Check sheet for the modelled part. Datum: model origin and axes. Units: mm. Face numbers are marked on the shaded views. A direction names the side the tool comes from. Give positions to 0.01 mm unless a question says otherwise; leave off trailing zeros. Write each loop counter-clockwise with the first axis right and the second up, starting at its lowest first coordinate (ties: lowest second). Pieces come first, ordered by that corner, then holes. Notation, with made-up numbers: (-37.75, 6.25) -> (5.25, 6.25) arc R32 cw to (5.25, 44.25) -> close; hole circle Ø11 at (-25.75, 16.5). An arc over 180 degrees is marked (long way). Use a Markdown table: item, result. Add a question column.
1. Cross-section at C-C (z = 12.5). Enter the section's corners in (x, y), then the cut area to 3 significant figures.
2. Cross-section at B-B (x = 15). Enter the section's corners in (y, z).
3. Scan lines: probe 1 along X at (y, z) = (22, 12.5); probe 2 along Y at (x, z) = (-5, 43); probe 3 along Y at (x, z) = (13, 44.5). Record each from-to range of solid material in increasing order. Write a range as [from, to].
4. Cross-section at A-A (z = 29). Enter the section's corners in (x, y).
5. Cross-section at D-D (x = -3). Enter the section's corners in (y, z).
6. Gauge pin test, flat ends, axial feed: P1, Ø7, axis at y = 15, z = 16.5, coming from the -X side; P2, Ø5, axis at x = -6, z = 8, coming from the +Y side; P3, Ø5, axis at x = 3, y = -2.5, coming from the +Z side; P4, Ø7.5, axis at y = 8.5, z = 54.5, coming from the +X side. Record the tip position at first contact, or that the pin passes through.
7. Release check for a two-part mould opening along Y. For the marked faces 6, 7 and 8 record: released by +Y, released by -Y, zero draft, split by the parting line, or undercut.
8. Set-up check for the marked faces 1, 2, 3, 4 and 5: record each of +Z, -Z, +X, -X, +Y, -Y from which the full face is reachable in a straight line by a thin tool's end or side.
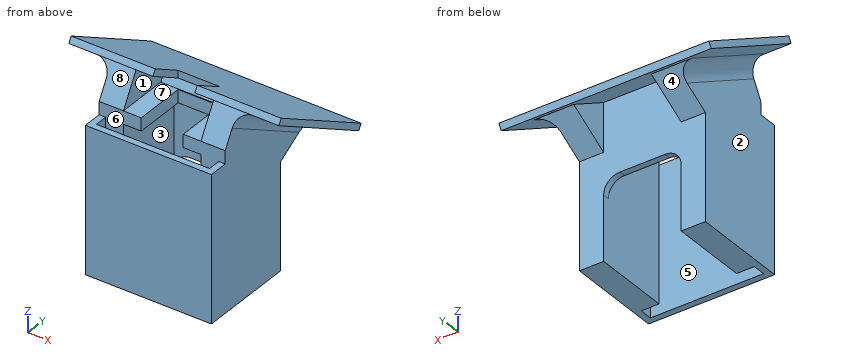
from build123d import *

# Parameters (mm, degrees)
EXTRUDE_1_DEPTH          = 45
EXTRUDE_2_DEPTH          = 4
SKETCH_3_W               = 24
SKETCH_3_H               = 2
CUT_EXTRUDE_1_DEPTH      = 25
SKETCH_5_W               = 40
SKETCH_5_H               = 65
EXTRUDE_3_DEPTH          = 1
CUT_EXTRUDE_2_DEPTH      = 72.51497427
CUT_EXTRUDE_2_DEPTH_BACK = 72.51497427
SKETCH_6_W               = 13
SKETCH_6_H               = 16
EXTRUDE_6_DEPTH          = 2
EXTRUDE_7_DEPTH          = 2
EXTRUDE_8_DEPTH          = 2
EXTRUDE_9_DEPTH          = 2
FILLET_1_R               = 5
EXTRUDE_10_DEPTH         = 5.5
EXTRUDE_11_DEPTH         = 5.5
SKETCH_18_W              = 24
SKETCH_18_H              = 5
EXTRUDE_13_DEPTH         = 3
FILLET_2_R               = 5


with BuildPart() as part:
    # Sketch 1 → Extrude 1 (new body)
    with BuildSketch(Plane.XY):
        Polygon((-14, 24), (-14, 2), (-19.5, 2), (-19.5, -6), (19.5, -6), (19.5, 2), (14, 2), (14, 24), align=None)
        Polygon((-12, 0), (-12, 22), (12, 22), (12, 0), (17.5, 0), (17.5, -4), (-17.5, -4), (-17.5, 0), align=None, mode=Mode.SUBTRACT)
    extrude(amount=EXTRUDE_1_DEPTH)

    # Sketch 2 → Extrude 2 (add)
    with BuildSketch(Plane.XY.offset(45)):
        Polygon((-14, 24), (-14, 0), (-6.5, 0), (-6.5, 16), (6.5, 16), (6.5, 0), (14, 0), (14, 24), align=None)
    extrude(amount=EXTRUDE_2_DEPTH)

    # Sketch 3 → Cut-Extrude 1 (cut)
    with BuildSketch(Plane(origin=(0, 0, 0), x_dir=(-1, 0, 0), z_dir=(0, 0, -1))):
        with Locations((0, 23)):
            Rectangle(SKETCH_3_W, SKETCH_3_H)
    extrude(amount=-CUT_EXTRUDE_1_DEPTH, mode=Mode.SUBTRACT)



with BuildPart() as body_2:
    # Sketch 5 → Extrude 3 (new, symmetric)
    with BuildSketch(Plane(origin=(0, 27.217622393, 47.142304845), x_dir=(0, -0.8660254037844413, 0.4999999999999954), z_dir=(0, 0.4999999999999954, 0.8660254037844413))):
        with Locations((5, 0)):
            Rectangle(SKETCH_5_W, SKETCH_5_H)
    extrude(amount=EXTRUDE_3_DEPTH, both=True)

    # Sketch 6 → Cut-Extrude 2 (cut, two sides: drawn at the far end of the back side and taken through both)
    with BuildSketch(Plane.XY.offset(49).offset(-CUT_EXTRUDE_2_DEPTH_BACK)):
        with Locations((0, 8)):
            Rectangle(SKETCH_6_W, SKETCH_6_H)
    extrude(amount=CUT_EXTRUDE_2_DEPTH + CUT_EXTRUDE_2_DEPTH_BACK, mode=Mode.SUBTRACT)


with BuildPart() as part_1:
    add(part.part)

    add(body_2.part)  # Extrude 6 merges body 2
    # Sketch 11 → Extrude 6 (add)
    with BuildSketch(Plane.ZY.offset(14)):
        Polygon((40.345299462, 36.990381057), (32.845299462, 24), (47.845299462, 24), align=None)
    extrude(amount=-EXTRUDE_6_DEPTH)

    # Sketch 12 → Extrude 7 (add)
    with BuildSketch(Plane(origin=(14, 0, 0), x_dir=(0, 0, -1), z_dir=(1, 0, 0))):
        Polygon((-47.845299462, 24), (-32.845299462, 24), (-40.345299462, 36.990381057), align=None)
    extrude(amount=-EXTRUDE_7_DEPTH)

    # Sketch 13 → Extrude 8 (add)
    with BuildSketch(Plane.ZY.offset(14)):
        Polygon((49, 22), (49, 0), (58.526279442, 5.5), align=None)
    extrude(amount=-EXTRUDE_8_DEPTH)

    # Sketch 14 → Extrude 9 (add)
    with BuildSketch(Plane(origin=(14, 0, 0), x_dir=(0, 0, -1), z_dir=(1, 0, 0))):
        Polygon((-49, 22), (-49, 0), (-58.526279442, 5.5), align=None)
    extrude(amount=-EXTRUDE_9_DEPTH)

    # Fillet 1
    fillet_1_edges = [part_1.edges().sort_by_distance(p)[0] for p in [
        (12, 23, 25),
        (-12, 23, 25),
    ]]
    fillet(fillet_1_edges, radius=FILLET_1_R)

    # Sketch 16 → Extrude 10 (add)
    with BuildSketch(Plane.ZY.offset(14)):
        Polygon((0, 24), (0, 2), (45, 2), (45, 0), (49, 0), (58.526279442, 5.5), (40.345299462, 36.990381057), (32.845299462, 24), align=None)
    extrude(amount=EXTRUDE_10_DEPTH)

    # Sketch 17 → Extrude 11 (add)
    with BuildSketch(Plane(origin=(14, 0, 0), x_dir=(0, 0, -1), z_dir=(1, 0, 0))):
        Polygon((0, 24), (0, 2), (-45, 2), (-45, 0), (-49, 0), (-58.526279442, 5.5), (-40.345299462, 36.990381057), (-32.845299462, 24), align=None)
    extrude(amount=EXTRUDE_11_DEPTH)

    # Sketch 18 → Extrude 13 (add)
    with BuildSketch(Plane(origin=(0, 26.717622393, 46.276279442), x_dir=(-1, 0, 0), z_dir=(0, -0.4999999999999954, -0.8660254037844414))):
        with Locations((0, -7.947441117)):
            Rectangle(SKETCH_18_W, SKETCH_18_H)
    extrude(amount=EXTRUDE_13_DEPTH)

    # Fillet 2
    fillet_2_edges = [part_1.edges().sort_by_distance(p)[0] for p in [
        (-19.5, 21.245190528, 49.435789452),
        (19.5, 21.245190528, 49.435789452),
    ]]
    fillet(fillet_2_edges, radius=FILLET_2_R)


solid = part_1.part
Worked answers:
| question | item | result |
|---|---|---|
| 1 | outline | (-19.5, -6) -> (19.5, -6) -> (19.5, 24) -> (12, 24) -> (12, 0) -> (17.5, 0) -> (17.5, -4) -> (-17.5, -4) -> (-17.5, 0) -> (-12, 0) -> (-12, 24) -> (-19.5, 24) -> close |
| 1 | area | 454 mm² |
| 2 | outline | (-6, 0) -> (-4, 0) -> (-4, 45) -> (-6, 45) -> close; (0, 0) -> (24, 0) -> (24, 32.85) -> (36.99, 40.35) -> (39.71, 38.78) -> (40.71, 40.51) -> (6.07, 60.51) -> (5.07, 58.78) -> (5.5, 58.53) -> (0, 49) -> close |
| 3 | probe 1 | x = [-19.5, -12], [12, 19.5] |
| 3 | probe 2 | y = [-6, -4], [22, 24], [32.39, 36.39] |
| 3 | probe 3 | y = [-6, -4], [0, 33.79] |
| 4 | outline | (-19.5, -6) -> (19.5, -6) -> (19.5, 24) -> (-19.5, 24) -> close; hole (-17.5, -4) -> (17.5, -4) -> (17.5, 0) -> (12, 0) -> (12, 22) -> (-12, 22) -> (-12, 0) -> (-17.5, 0) -> close |
| 5 | outline | (-6, 0) -> (-4, 0) -> (-4, 45) -> (-6, 45) -> close; (16, 45) -> (22, 45) -> (22, 25) -> (24, 25) -> (24, 47.85) -> (39.71, 38.78) -> (40.71, 40.51) -> (16, 54.77) -> (16, 52.46) -> (17.67, 51.5) -> (16.23, 49) -> (16, 49) -> close |
| 6 | P1 | stops at x = -19.5 |
| 6 | P2 | stops at y = -4 |
| 6 | P3 | stops at z = 45 |
| 6 | P4 | stops at x = 32.5 |
| 7 | face 6 | undercut |
| 7 | face 7 | zero draft |
| 7 | face 8 | released by -Y |
| 8 | face 1 | -Y |
| 8 | face 2 | -Z, -X, -Y |
| 8 | face 3 | -Z |
| 8 | face 4 | -Z, +X, -X |
| 8 | face 5 | +Z, -Z |
